Part model, mm, in its own coordinate system. A direction names the side the tool comes from. Round coordinates to 2 decimals unless told otherwise and drop trailing zeros. Write each loop counter-clockwise with the first axis right and the second up, starting at its lowest first coordinate (ties: lowest second). Pieces come first, ordered by that corner, then holes.
from build123d import *

# Parameters (mm, degrees)
SKETCH1_W                   = 25.4
SKETCH1_H                   = 66.675
BOSS_EXTRUDE1_DEPTH         = 9.525
TAP_DRILL_FOR_1_4_20_TAP1_D = 5.1054
SKETCH4_W                   = 3.175
SKETCH4_H                   = 57.15
CUT_EXTRUDE1_DEPTH          = 64.261426833
F_8_0_8_DIAMETER_HOLE1_D    = 8
CHAMFER1_SIZE               = 7.62
CUT_EXTRUDE2_DEPTH          = 86.959863454
CHAMFER2_SIZE               = 6.35
FILLET1_DEPTH               = 6.35
CHAMFER3_SIZE               = 3.175


with BuildPart() as part:
    # Sketch1 → Boss-Extrude1 (new body)
    with BuildSketch(Plane.XY):
        with Locations((50.8, 23.8125)):
            Rectangle(SKETCH1_W, SKETCH1_H)
    extrude(amount=BOSS_EXTRUDE1_DEPTH)

    # Tap Drill for 1/4-20 Tap1 (through all)
    with Locations(Plane(origin=(0, 0, 0), x_dir=(-1, 0, 0), z_dir=(0, 0, -1))):
        with Locations((-50.8, 47.625), (-50.8, 9.525)):
            Hole(TAP_DRILL_FOR_1_4_20_TAP1_D / 2)

    # Sketch4 → Cut-Extrude1 (cut, through all)
    with BuildSketch(Plane(origin=(63.5, 0, 0), x_dir=(0, 0, -1), z_dir=(1, 0, 0))):
        with Locations((-7.9375, 28.575)):
            Rectangle(SKETCH4_W, SKETCH4_H)
    extrude(amount=-CUT_EXTRUDE1_DEPTH, mode=Mode.SUBTRACT)

    # Ø8.0 (8) Diameter Hole1 (through all)
    with Locations(Plane(origin=(0, 0, 0), x_dir=(-1, 0, 0), z_dir=(0, 0, -1))):
        with Locations((-50.732643015, -4.7625)):
            Hole(F_8_0_8_DIAMETER_HOLE1_D / 2)

    # Chamfer1
    chamfer1_edges = [part.edges().sort_by_distance(p)[0] for p in [
        (63.5, -9.525, 4.7625),
        (38.1, -9.525, 4.7625),
    ]]
    chamfer(chamfer1_edges, length=CHAMFER1_SIZE)

    # Sketch7 → Cut-Extrude2 (cut, through all)
    with BuildSketch(Plane(origin=(0, 0, 0), x_dir=(-1, 0, 0), z_dir=(0, 0, -1))):
        Polygon((-44.45, 15.875), (-21.210032305, 15.875), (-21.210032305, 64.752426372), (-78.308679705, 64.752426372), (-78.308679705, 15.875), (-57.15, 15.875), (-57.15, 53.975), (-44.45, 53.975), align=None)
    extrude(amount=-CUT_EXTRUDE2_DEPTH, mode=Mode.SUBTRACT)

    # Chamfer2
    chamfer2_edges = [part.edges().sort_by_distance(p)[0] for p in [
        (38.1, 15.875, 3.175),
        (63.5, 15.875, 3.175),
    ]]
    chamfer(chamfer2_edges, length=CHAMFER2_SIZE - 0.0001)  # a hair under: the kernel refuses the full size

    # Fillet1: read off the stored shape, not the designer's step
    # Fillet1 outline → Fillet1 (add)
    with BuildSketch(Plane.XY):
        with BuildLine():
            ThreePointArc((44.45, 17.190128061), (44.208317516, 15.975108163), (43.52006403, 14.94506403))
            Line((43.52006403, 14.94506403), (44.45, 15.875))
            Line((44.45, 15.875), (44.45, 17.190128061))
        make_face()
        with BuildLine():
            ThreePointArc((58.07993597, 14.94506403), (57.391682484, 15.975108163), (57.15, 17.190128061))
            Line((57.15, 17.190128061), (57.15, 15.875))
            Line((57.15, 15.875), (58.07993597, 14.94506403))
        make_face()
    extrude(amount=FILLET1_DEPTH)

    # Chamfer3
    chamfer3_edges = [part.edges().sort_by_distance(p)[0] for p in [
        (57.15, 53.975, 3.175),
        (44.45, 53.975, 3.175),
    ]]
    chamfer(chamfer3_edges, length=CHAMFER3_SIZE)


solid = part.part
Q1. Saw through at C-C, the plane z = 5.5. Give the number of separate pieces and of enclosed holes in the cut face, and give its area (3 significant figures).
Q2. Saw through at D-D, the plane x = 62. Write the cut outline in (y, z) (3 decimals), and give its area (3 significant figures).
Q3. Saw through at B-B, the plane x = 50.8. Write the cut outline in (y, z) (3 decimals).
Q4. Drop flat-ended pins along their axis: P1, Ø4.5, axis at x = 50.8, y = 47.625, coming from the -Z side (3 decimals); P2, Ø1, axis at x = 44, z = 8.5, coming from the -Y side (3 decimals); P3, Ø1.9, axis at y = 27, z = 4, coming from the +X side; P4, Ø8, axis at x = 51, y = 8, coming from the +Z side. Give the stop position or say it passes through.
Q5. Tool access for faces 4 (the flat face through (57.15, 34, 3)), 5 (the cylindrical face through (46.737, -4.587, 4.829)): list every direction of +Z, -Z, +X, -X, +Y, -Y with a clear straight run to the whole face (end or side of a thin tool).
Q6. Saw through at A-A, the plane y = 11.5. Write the cut outline in (x, z), and give its area (3 significant figures).
Q7. Wall check: line 1 (Y direction, x = 50.8, z = 2.5) (3 decimals); line 2 (Y direction, x = 50, z = 1) (3 decimals); line 3 (X direction, y = 20.5, z = 6.25). Give the ranges that are in metal, low to high.
Q8. Two-plate mould, pull along X, no slides. Class faces 1 (the flat face through (51, 21, 6.35)), 2 (the cylindrical face through (50.247, 45.133, 3.219)), 3 (the flat face through (41.963, -5.768, 4.696)): released by +X, released by -X, zero draft, split by the parting line, or undercut.
Computed:
1. separate pieces: 1
1. enclosed holes: 3
1. area: 930 mm2
2. outline: (-3.405, 0) - (11.025, 0) - (11.025, 6.35) - (0, 6.35) - (0, 9.525) - (-3.405, 9.525) - close
2. area: 102 mm2
3. outline: (-9.525, 0) - (-8.762, 0) - (-8.762, 9.525) - (-9.525, 9.525) - close; (-0.763, 0) - (6.972, 0) - (6.972, 6.35) - (0, 6.35) - (0, 9.525) - (-0.763, 9.525) - close; (12.078, 0) - (45.072, 0) - (45.072, 6.35) - (12.078, 6.35) - close; (50.178, 0) - (53.975, 0) - (53.975, 6.35) - (50.178, 6.35) - close
4. P1: passes through
4. P2: stops at y = -8.305
4. P3: stops at x = 57.15
4. P4: stops at z = 6.35
5. face 4: +Z, -Z, +X, +Y
5. face 5: +Z, -Z
6. outline: (40.07, 0) - (49.18, 0) - (49.18, 6.35) - (40.07, 6.35) - close; (52.42, 0) - (61.53, 0) - (61.53, 6.35) - (52.42, 6.35) - close
6. area: 116 mm2
7. line 1: y = -9.525 to -8.762, -0.763 to 6.972, 12.078 to 45.072, 50.178 to 53.975
7. line 2: y = -9.525 to -8.695, -0.83 to 7.101, 11.949 to 45.201, 50.049 to 53.975
7. line 3: x = 44.45 to 57.15
8. face 1: zero draft
8. face 2: undercut
8. face 3: released by -X
